Source: CAD feature listing. Evaluate the final solid. Frame: model axes, mm. Face numbers are marked on the shaded views. A direction names the side the tool comes from. Round coordinates to 2 decimals unless told otherwise and drop trailing zeros. Order: outer loops, then holes, each group sorted by start corner. A loop starts at its lowest first (then second) coordinate and runs counter-clockwise, first axis right, second up. Notation, with made-up numbers: (23.5, 88) -> (41.5, 88) arc R26 cw to (41.5, 115) -> close; hole circle Ø8 at (21.5, -2.75). An arc over 180 degrees is marked (long way). Use a Markdown table: item, result. Add a question column.
Autodesk Inventor part; units mm, degrees
ref_plane "YZ Plane" through (0, 0, 0) normal (1, 0, 0) x (0, 1, 0)
ref_plane "XZ Plane" through (0, 0, 0) normal (0, 1, 0) x (-1, 0, 0)
ref_plane "XY Plane" through (0, 0, 0) normal (0, 0, 1) x (1, 0, 0)
sketch "Sketch1" plane through (0, 0, 0) normal (0, 0, 1) x (1, 0, 0)
  line L0 (-2.8403, 5.136) -> (-4.6718, 3.4343)
  line L1 (-4.2463, -3.182) -> (-4.6718, 3.4343)
  line L2 (-4.2463, -3.182) -> (3.182, -3.182)
  line L3 (3.182, -3.182) -> (3.182, 4.3178)
  line L4 (-2.8403, 5.136) -> (3.182, 4.3178)
  circle A0 centre (0, 0) radius 1.2484
  circle A1 centre (0, 3) radius 0.7934
  circle A2 centre (-1.875, -1.75) radius 0.7934
  circle A3 centre (1.875, -1.75) radius 0.7934
  line L5 (-4.569, 3.3933) -> (-2.8069, 5.0305)
  line L6 (-2.8069, 5.0305) -> (3.082, 4.2305)
  line L7 (3.082, 4.2305) -> (3.082, -3.082)
  line L8 (3.082, -3.082) -> (-4.1525, -3.082)
  line L9 (-4.1525, -3.082) -> (-4.569, 3.3933)
  dimension "d0" = 0.1
extrude "Extrusion1" add sketch "Sketch1" along normal blind 1 contours L5 L6 L7 L8 L9
sketch "Sketch2" plane through (0, 0, 1) normal (0, 0, 1) x (1, 0, 0)
  line L0 (-2.8403, 5.136) -> (-4.6718, 3.4343)
  line L1 (-4.2463, -3.182) -> (-4.6718, 3.4343)
  line L2 (-4.2463, -3.182) -> (3.182, -3.182)
  line L3 (3.182, -3.182) -> (3.182, 4.3178)
  line L4 (-2.8403, 5.136) -> (3.182, 4.3178)
  circle A0 centre (0, 0) radius 1.2484
  circle A1 centre (0, 3) radius 0.7934
  circle A2 centre (-1.875, -1.75) radius 0.7934
  circle A3 centre (1.875, -1.75) radius 0.7934
  line L5 (-4.569, 3.3933) -> (-2.8069, 5.0305)
  line L6 (-2.8069, 5.0305) -> (3.082, 4.2305)
  line L7 (3.082, 4.2305) -> (3.082, -3.082)
  line L8 (3.082, -3.082) -> (-4.1525, -3.082)
  line L9 (-4.1525, -3.082) -> (-4.569, 3.3933)
  circle A4 centre (0, 3) radius 0.375
  circle A5 centre (1.875, -1.75) radius 0.375
  circle A6 centre (-1.875, -1.75) radius 0.375
  dimension "d3" = 0.1
  dimension "d4" = 1.5869
  dimension "d5" = 0.75
  dimension "d6" = 0.75
  dimension "d7" = 0.75
extrude "Extrusion2" add sketch "Sketch2" along normal blind 4.43 contours A1 | A2 | A3 | L5 L6 L7 L8 L9
sketch "Sketch3" plane through (0, 0, 5.43) normal (0, 0, 1) x (1, 0, 0)
  line L0 (-2.8403, 5.136) -> (-4.6718, 3.4343)
  line L1 (-4.2463, -3.182) -> (-4.6718, 3.4343)
  line L2 (-4.2463, -3.182) -> (3.182, -3.182)
  line L3 (3.182, -3.182) -> (3.182, 4.3178)
  line L4 (-2.8403, 5.136) -> (3.182, 4.3178)
  circle A0 centre (0, 0) radius 1.2484
  circle A1 centre (0, 3) radius 0.7934
  circle A2 centre (-1.875, -1.75) radius 0.7934
  circle A3 centre (1.875, -1.75) radius 0.7934
  line L5 (-4.569, 3.3933) -> (-2.8069, 5.0305)
  line L6 (-2.8069, 5.0305) -> (3.082, 4.2305)
  line L7 (3.082, 4.2305) -> (3.082, -3.082)
  line L8 (3.082, -3.082) -> (-4.1525, -3.082)
  line L9 (-4.1525, -3.082) -> (-4.569, 3.3933)
  circle A4 centre (0, 3) radius 0.375
  circle A5 centre (1.875, -1.75) radius 0.375
  circle A6 centre (-1.875, -1.75) radius 0.375
  dimension "d10" = 0.1
  dimension "d11" = 1.5869
  dimension "d12" = 0.75
  dimension "d13" = 0.75
  dimension "d14" = 0.75
extrude "Extrusion3" add sketch "Sketch3" along normal blind 1 contours A0 | A1 | A2 | A3 | L5 L6 L7 L8 L9
sketch "Sketch5" plane through (0, 0, 6.43) normal (0, 0, 1) x (1, 0, 0)
  circle A0 centre (0, 0) radius 1.2484
  circle A1 centre (0, 0) radius 2.1
  line L0 (5.5495, -5.5229) -> (-7.4793, -5.5229)
  line L1 (-7.4793, -5.5229) -> (-7.4793, 6.9136)
  line L2 (-7.4793, 6.9136) -> (5.5495, 6.9136)
  line L3 (5.5495, 6.9136) -> (5.5495, -5.5229)
  dimension "d18" = 4.2
extrude "Extrusion4" cut sketch "Sketch5" against normal blind 4 contours L0 L1 L2 L3
sketch "Sketch6" plane through (0, 0, 0) normal (0, 0, -1) x (-1, 0, 0)
  circle A0 centre (0, 0) radius 1.2484
  circle A1 centre (0, 3) radius 0.7934
  circle A2 centre (1.875, -1.75) radius 0.7934
  circle A3 centre (-1.875, -1.75) radius 0.7934
  line L0 (4.569, 3.3933) -> (2.8069, 5.0305)
  line L1 (2.8069, 5.0305) -> (-3.082, 4.2305)
  line L2 (-3.082, 4.2305) -> (-3.082, -3.082)
  line L3 (-3.082, -3.082) -> (4.1525, -3.082)
  line L4 (4.1525, -3.082) -> (4.569, 3.3933)
extrude "Extrusion5" add sketch "Sketch6" along normal blind 0.15
chamfer "Chamfer1" distance 0.2 angle 45 4 edges at (-1.0816, -1.75, -0.15) (2.6684, -1.75, -0.15) (0.7934, 3, -0.15) (1.2484, 0, -0.15)
properties part number "Cover"
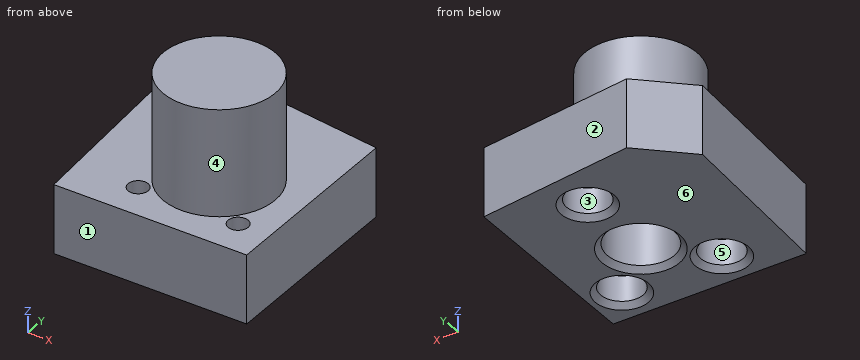
1) Section C-C on z = 5.25. Output: boundary loops of the cut face in (x, y).
2) Section B-B on y = 1.75. Output: boundary loops of the cut face in (x, z).
3) Line query: probe 1 along X at (y, z) = (-1.5, 2); probe 2 along Y at (x, z) = (0, 0.35); probe 3 along X at (y, z) = (-1.75, 0.6). Output: solid intervals per line, ascending. Write a range as from..to.
4) Section A-A on z = 1.25. Count the separate pieces of the cut face and the enclosed holes in it, then the cut area to 3 significant figures.
5) First-contact query: pin 1 Ø1.4 at (x, y) = (1.875, -1.75) entering from +Z; pin 2 Ø3 at (x, z) = (-1, 0.5) entering from +Y; pin 3 Ø1.5 at (x, y) = (0, 0) entering from -Z; pin 4 Ø1.5 at (y, z) = (-0.5, 3.5) entering from +X. Flat tips, straight axial feed; report the tip coordinate or a pass-through.
6) Reachability of the marked faces 4, 5 and 6 from +Z, -Z, +X, -X, +Y, -Y: full face, straight path, thin tool, end or side. Return the list, or none.
7) Draft query along Y for the marked faces 1, 2 and 3. Return one class per face: pulls with the +Y half, pulls with the -Y half, needs draft (parallel to the pull), parting line crosses it, or undercut.
Conclusion:
| question | item | result |
|---|---|---|
| 1 | outline | circle Ø4.2 at (0, 0); hole circle Ø2.5 at (0, 0) |
| 2 | outline | (-4.46, -0.15) -> (3.08, -0.15) -> (3.08, 2.43) -> (1.16, 2.43) -> (1.16, 6.43) -> (-1.16, 6.43) -> (-1.16, 2.43) -> (-4.46, 2.43) -> close |
| 3 | probe 1 | x = -4.25..-2.15, -1.6..1.6, 2.15..3.08 |
| 3 | probe 2 | y = -3.08..-1.25, 1.25..2.21, 3.79..4.65 |
| 3 | probe 3 | x = -4.24..-2.67, -1.08..1.08, 2.67..3.08 |
| 4 | separate pieces | 1 |
| 4 | enclosed holes | 4 |
| 4 | area | 50.7 mm^2 |
| 5 | pin 1 | stops at z = 6.43 |
| 5 | pin 2 | stops at y = 4.99 |
| 5 | pin 3 | stops at z = 5.43 |
| 5 | pin 4 | stops at x = 2.1 |
| 6 | face 4 | +Z |
| 6 | face 5 | -Z |
| 6 | face 6 | -Z, +X, -X, +Y, -Y |
| 7 | face 1 | pulls with the -Y half |
| 7 | face 2 | pulls with the +Y half |
| 7 | face 3 | undercut |
